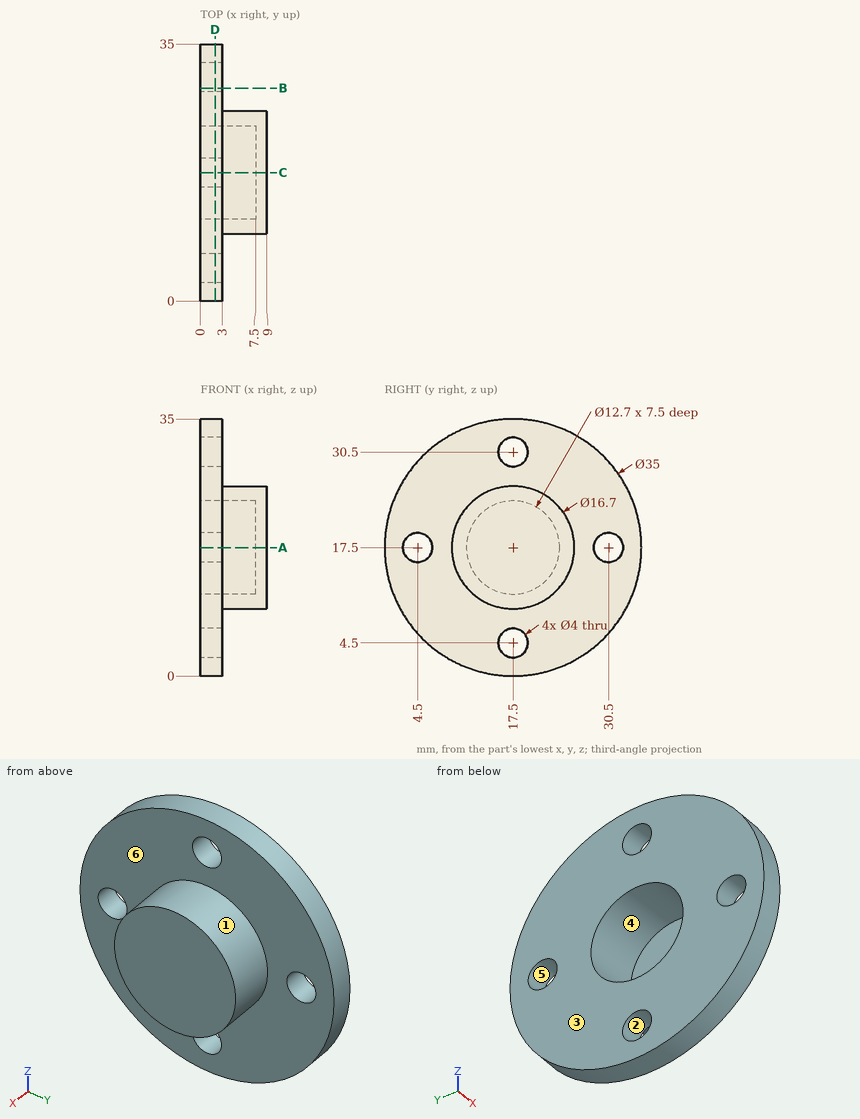
The drawing under review shows one solid part. Ordinate dimensions are in mm from its lowest x, y, z. A direction names the side the tool comes from. Coordinates: 2 decimals unless noted, no trailing zeros. Loops run counter-clockwise (first coordinate to the right, second up) from the corner with the lowest first, then second, coordinate; pieces in that order, holes last.
Item 1: For the marked faces 4, 5 and 6, list the 3-axis set-ups (+Z, -Z, +X, -X, +Y, -Y) from which the entire face can be reached by the end or side of a thin tool; tool diameter is ignored.
Completed:
face 4: -X
face 5: +X, -X
face 6: +X
Item 2: Add section D-D (x = 2). Write out the cut boundary in (y, z).
Completed:
outline: circle Ø35 at (17.5, 17.5); hole circle Ø4 at (4.5, 17.5); hole circle Ø12.7 at (17.5, 17.5); hole circle Ø4 at (17.5, 4.5); hole circle Ø4 at (17.5, 30.5); hole circle Ø4 at (30.5, 17.5)
Item 3: Clearance check with flat-ended pins moving along their axes: pin 1 (14.5 mm diameter, centred on y = 17.5, z = 17.5, fed in from -X); pin 2 (5 mm diameter, centred on y = 4.5, z = 17.5, fed in from +X); pin 3 (1 mm diameter, centred on x = 2.5, y = 21, fed in from +Z); pin 4 (2 mm diameter, centred on x = 2.5, y = 27, fed in from -Z). State where each tip first meets the part, or that it passes through.
Completed:
pin 1: stops at x = 0
pin 2: stops at x = 3
pin 3: stops at z = 34.74
pin 4: stops at z = 2.2
Item 4: Wall thickness on L1, parallel to Z at x = 1, y = 17.5; L2, parallel to Z at x = 3.25, y = 17.5; L3, parallel to X at y = 20, z = 15: over which ranges is each line inside the solid? List them lowest first.
Completed:
L1: z = 0 to 2.5, 6.5 to 11.15, 23.85 to 28.5, 32.5 to 35
L2: z = 9.15 to 11.15, 23.85 to 25.85
L3: x = 7.5 to 9
Item 5: Draft analysis for pull direction Z (two halves, no side actions). For the marked faces 1, 2 and 3, state which applies: pulls with the +Z half, pulls with the -Z half, needs draft (parallel to the pull), parting line crosses it, or undercut.
Completed:
face 1: parting line crosses it
face 2: undercut
face 3: needs draft
Item 6: Add section B-B (y = 29). Write out the cut boundary in (x, z), and give its area (3 significant figures).
Completed:
outline: (0, 4.31) - (3, 4.31) - (3, 16.18) - (0, 16.18) - close; (0, 18.82) - (3, 18.82) - (3, 30.69) - (0, 30.69) - close
area: 71.2 mm2
Item 7: Add section A-A (z = 17.5). Write out the cut boundary in (x, y).
Completed:
outline: (0, 0) - (3, 0) - (3, 2.5) - (0, 2.5) - close; (0, 6.5) - (3, 6.5) - (3, 9.15) - (9, 9.15) - (9, 25.85) - (3, 25.85) - (3, 28.5) - (0, 28.5) - (0, 23.85) - (7.5, 23.85) - (7.5, 11.15) - (0, 11.15) - close; (0, 32.5) - (3, 32.5) - (3, 35) - (0, 35) - close
